Could you check a few things on this model? Use its own coordinates, in mm. Round coordinates to 2 decimals unless told otherwise and drop trailing zeros. Write each loop counter-clockwise with the first axis right and the second up, starting at its lowest first coordinate (ties: lowest second). Pieces come first, ordered by that corner, then holes. Notation, with made-up numbers: M 21.25,56.25 L 51.25,56.25 A9 ccw 51.25,62.25 Z; hole C -14,7.25 d1. An arc over 180 degrees is marked long. One line per item, written item: value. Start each with the question number.
(1) I want a section at D-D on x = 1.85. Please give me the cut outline in (y, z).
(2) I want a section at B-B on y = 7. Please give me the cut outline in (x, z), and give its area (3 significant figures).
(3) I want a section at A-A on z = -10. Please give me the cut outline in (x, y).
(4) I want a section at C-C on y = 22. Please give me the cut outline in (x, z).
(5) If I drill on L1, parallel to Y at x = 0.6, z = -10; L2, parallel to Z at x = 0.7, y = 6.5; L3, parallel to Y at x = 1.6, z = -84, over which ranges is the centre line in solid material (lowest first)?
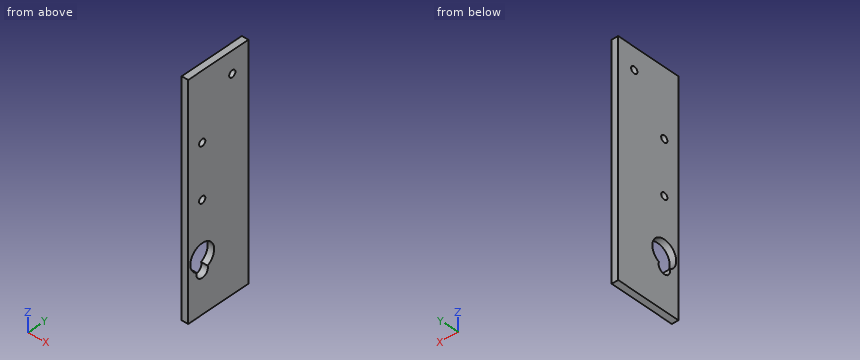
```python
from build123d import *

# Parameters (mm, degrees)
SKIZZE1_W                       = 105
SKIZZE1_H                       = 30
AUFSATZ_LINEAR_AUSTRAGEN1_DEPTH = 3
SKIZZE2_R                       = 1.55
BOHRUNGEN_DEPTH                 = 110.242848736
SCHNITT_LINEAR_AUSTRAGEN4_DEPTH = 3


with BuildPart() as part:
    # Skizze1 → Aufsatz-Linear austragen1 (new body)
    with BuildSketch(Plane(origin=(0, 0, 0), x_dir=(0, 0, -1), z_dir=(1, 0, 0))):
        with Locations((52.5, 15)):
            Rectangle(SKIZZE1_W, SKIZZE1_H)
    extrude(amount=AUFSATZ_LINEAR_AUSTRAGEN1_DEPTH)

    # Skizze2 → Bohrungen (cut, through all)
    with BuildSketch(Plane(origin=(3, 0, 0), x_dir=(0, 0, -1), z_dir=(1, 0, 0))):
        with Locations((10, 22)):
            Circle(SKIZZE2_R)
        with Locations((31, 7)):
            Circle(SKIZZE2_R)
        with Locations((55.59187467, 7)):
            Circle(SKIZZE2_R)
        with Locations((80.183749339, 7)):
            Circle(SKIZZE2_R)
    extrude(amount=-BOHRUNGEN_DEPTH, mode=Mode.SUBTRACT)

    # Skizze7 → Schnitt-Linear austragen4 (cut)
    with BuildSketch(Plane(origin=(0, 0, 0), x_dir=(0, 0, -1), z_dir=(1, 0, 0))):
        with BuildLine():
            ThreePointArc((85.483749339, 9.704163457), (74.233749339, 7), (85.483749339, 4.295836543))
            ThreePointArc((85.483749339, 4.295836543), (89.233749339, 7), (85.483749339, 9.704163457))
        make_face()
    extrude(amount=SCHNITT_LINEAR_AUSTRAGEN4_DEPTH, mode=Mode.SUBTRACT)


solid = part.part
```
Found:
1. outline: M 0,-105 L 30,-105 L 30,0 L 0,0 Z; hole M 4.3,-85.48 A2.85 ccw long 9.7,-85.48 A5.95 ccw long Z; hole C 7,-55.59 d3.1; hole C 7,-31 d3.1; hole C 22,-10 d3.1
2. outline: M 0,-105 L 3,-105 L 3,-89.23 L 0,-89.23 Z; M 0,-74.23 L 3,-74.23 L 3,-57.14 L 0,-57.14 Z; M 0,-54.04 L 3,-54.04 L 3,-32.55 L 0,-32.55 Z; M 0,-29.45 L 3,-29.45 L 3,0 L 0,0 Z
2. area: 251 mm²
3. outline: M 0,0 L 3,0 L 3,20.45 L 0,20.45 Z; M 0,23.55 L 3,23.55 L 3,30 L 0,30 Z
4. outline: M 0,-105 L 3,-105 L 3,-11.55 L 0,-11.55 Z; M 0,-8.45 L 3,-8.45 L 3,0 L 0,0 Z
5. L1: y = 0 to 20.45, 23.55 to 30
5. L2: z = -105 to -89.19, -74.25 to -57.06, -54.12 to -32.47, -29.53 to 0
5. L3: y = 0 to 2.44, 11.56 to 30
